from build123d import *

# Parameters (mm, degrees)
SHELL1_T       = -3.175
CHAMFER1_SIZE  = 0.762
CHAMFER1_SIZE2 = 0.885503909


with BuildPart() as part:
    # Sketch1 → Revolve1 (revolve)
    with BuildSketch(Plane(origin=(0, 0, 0), x_dir=(0, 0, -1), z_dir=(1, 0, 0)), mode=Mode.PRIVATE) as revolve1_sk:
        Polygon((0, 0), (41.275, 0), (42.9514969, 12.7), (0, 12.7), align=None)
    revolve(revolve1_sk.sketch.rotate(Axis((0, 0, 0), (0, -1, 0)), 180), axis=Axis((0, 0, 0), (0, -1, 0)))

    # Shell1
    shell1_openings = [part.faces().sort_by_distance(p)[0] for p in [
        (0, 12.7, 0),
    ]]
    offset(amount=SHELL1_T, openings=shell1_openings, kind=Kind.INTERSECTION)

    # Chamfer1
    chamfer1_edges = [part.edges().sort_by_distance(p)[0] for p in [
        (0, 0, -41.275),
    ]]
    chamfer1_side = [part.faces().sort_by_distance(p)[0] for p in [
        (0, 0, 0),
    ]]
    chamfer(chamfer1_edges, length=CHAMFER1_SIZE, length2=CHAMFER1_SIZE2, reference=chamfer1_side[0])


solid = part.part
Source: CAD feature listing. Evaluate the final solid. Frame: model axes, mm. Round coordinates to 2 decimals unless told otherwise and drop trailing zeros. Loops run counter-clockwise (first coordinate to the right, second up) from the corner with the lowest first, then second, coordinate; pieces in that order, holes last.
Q1. Section D-D, the plane y = 8.75. Return loops of the section in (x, z).
Q2. Ray query, line 1 (Z direction, x = 7, y = 9.25); line 2 (X direction, y = 4.5, z = 35); line 3 (X direction, y = 6.75, z = -10). Return the intervals inside material, ascending.
Q3. First-contact query: P1, Ø2, axis at x = -6, y = 6.5, coming from the +Z side; P2, Ø1, axis at x = 2.5, y = 6.5, coming from the +Z side; P3, Ø5, axis at x = -5, y = 5, coming from the -Z side. Flat tips, straight axial feed; report the tip coordinate or a pass-through.
Q4. Section C-C, the plane y = 4.25. Return loops of the section in (x, z).
Q5. Mould query, pull axis X, two halves, no side actions, for faces 1 (the face through (34.218, 3.771, 17.798)), 2 (the face through (38, 12.7, 13)), 3 (the face through (-1, 3.175, 1)), 4 (the face through (-41.135, 1.617, -5.401)). Classes: pulls with the +X half, pulls with the -X half, needs draft (parallel to the pull), parting line crosses it, or undercut.
Q6. Section B-B, the plane z = 0. Return loops of the section in (x, y) (1 decimal).
Q7. Section A-A, the plane x = 0. Return loops of the section in (y, z) (1 decimal).
Solutions:
1. outline: circle Ø84.86 at (0, 0); hole circle Ø78.46 at (0, 0)
2. line 1: z = -41.92 to -38.66, 38.66 to 41.92
2. line 2: x = -22.98 to -16.43, 16.43 to 22.98
2. line 3: x = -40.96 to -37.66, 37.66 to 40.96
3. P1: stops at z = 41.89
3. P2: stops at z = 42.13
3. P3: stops at z = -42.05
4. outline: circle Ø83.67 at (0, 0); hole circle Ø77.27 at (0, 0)
5. face 1: undercut
5. face 2: needs draft
5. face 3: undercut
5. face 4: parting line crosses it
6. outline: (-43, 12.7) - (-41.4, 0.9) - (-40.5, 0) - (40.5, 0) - (41.4, 0.9) - (43, 12.7) - (39.7, 12.7) - (38.5, 3.2) - (-38.5, 3.2) - (-39.7, 12.7) - close
7. outline: (0, -40.5) - (0.9, -41.4) - (12.7, -43) - (12.7, -39.7) - (3.2, -38.5) - (3.2, 38.5) - (12.7, 39.7) - (12.7, 43) - (0.9, 41.4) - (0, 40.5) - close
